The model under review builds one solid part; all positions refer to its coordinate system, in mm. Face numbers are marked on the shaded views. A direction names the side the tool comes from. Coordinates: 2 decimals unless noted, no trailing zeros. Write each loop counter-clockwise with the first axis right and the second up, starting at its lowest first coordinate (ties: lowest second). Pieces come first, ordered by that corner, then holes. Notation, with made-up numbers: M -38,66 L 13,66 A26 cw 13,101 Z; hole C -13,7.25 d8. An arc over 180 degrees is marked long. Answer as a JSON object with one key per item and string values.
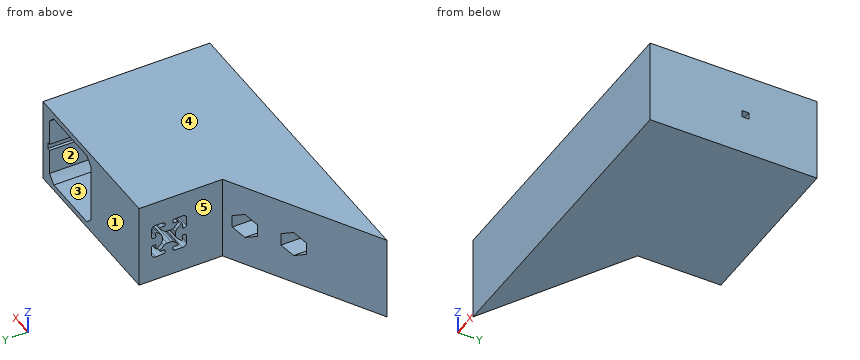
```python
from build123d import *

# Parameters (mm, degrees)
SKETCH1_W           = 35
SKETCH1_H           = 50
SKETCH1_W_2         = 62.5
BOSS_EXTRUDE1_DEPTH = 50
BOSS_EXTRUDE2_DEPTH = 50
CUT_EXTRUDE1_DEPTH  = 81
BOSS_EXTRUDE3_DEPTH = 50.006
SKETCH5_W           = 4
SKETCH5_H           = 4
CUT_EXTRUDE2_DEPTH  = 30
BOSS_EXTRUDE4_DEPTH = 50


with BuildPart() as part:
    # Sketch1 → Boss-Extrude1 (new body)
    # profile 1 of 2: a face of its own
    with BuildSketch(Plane.YZ):
        with Locations((80, 305)):
            Rectangle(SKETCH1_W, SKETCH1_H)
        with BuildLine():
            Line((76.1, 303.897755224), (76.1, 306.102244776))
            ThreePointArc((76.1, 306.102244776), (75.894474738, 307.135490044), (75.309188309, 308.011433085))
            Line((75.309188309, 308.011433085), (73.008308049, 310.312313346))
            ThreePointArc((73.008308049, 310.312313346), (72.488454457, 310.411010634), (72.206097787, 309.963502397))
            Line((72.206097787, 309.963502397), (72.280053987, 307.845673932))
            ThreePointArc((72.280053987, 307.845673932), (72.119231712, 307.415535218), (71.701359189, 307.225099738))
            Line((71.701359189, 307.225099738), (71.00178561, 307.20067009))
            ThreePointArc((71.00178561, 307.20067009), (70.213197967, 307.495510928), (69.864066254, 308.261610554))
            Line((69.864066254, 308.261610554), (69.701401098, 312.919731158))
            ThreePointArc((69.701401098, 312.919731158), (70.373654403, 314.626345597), (72.080268842, 315.298598902))
            Line((72.080268842, 315.298598902), (76.738389446, 315.135933746))
            ThreePointArc((76.738389446, 315.135933746), (77.504489072, 314.786802033), (77.79932991, 313.99821439))
            Line((77.79932991, 313.99821439), (77.774900262, 313.298640811))
            ThreePointArc((77.774900262, 313.298640811), (77.584464782, 312.880768288), (77.154326068, 312.719946013))
            Line((77.154326068, 312.719946013), (75.036497603, 312.793902213))
            ThreePointArc((75.036497603, 312.793902213), (74.588989366, 312.511545543), (74.687686654, 311.991691951))
            Line((74.687686654, 311.991691951), (76.988566915, 309.690811691))
            ThreePointArc((76.988566915, 309.690811691), (77.864509956, 309.105525262), (78.897755224, 308.9))
            Line((78.897755224, 308.9), (81.102244776, 308.9))
            ThreePointArc((81.102244776, 308.9), (82.135490044, 309.105525262), (83.011433085, 309.690811691))
            Line((83.011433085, 309.690811691), (85.312313346, 311.991691951))
            ThreePointArc((85.312313346, 311.991691951), (85.411010634, 312.511545543), (84.963502397, 312.793902213))
            Line((84.963502397, 312.793902213), (82.845673932, 312.719946013))
            ThreePointArc((82.845673932, 312.719946013), (82.415535218, 312.880768288), (82.225099738, 313.298640811))
            Line((82.225099738, 313.298640811), (82.20067009, 313.99821439))
            ThreePointArc((82.20067009, 313.99821439), (82.495510928, 314.786802033), (83.261610554, 315.135933746))
            Line((83.261610554, 315.135933746), (87.919731158, 315.298598902))
            ThreePointArc((87.919731158, 315.298598902), (89.626345597, 314.626345597), (90.298598902, 312.919731158))
            Line((90.298598902, 312.919731158), (90.135933746, 308.261610554))
            ThreePointArc((90.135933746, 308.261610554), (89.786802033, 307.495510928), (88.99821439, 307.20067009))
            Line((88.99821439, 307.20067009), (88.298640811, 307.225099738))
            ThreePointArc((88.298640811, 307.225099738), (87.880768288, 307.415535218), (87.719946013, 307.845673932))
            Line((87.719946013, 307.845673932), (87.793902213, 309.963502397))
            ThreePointArc((87.793902213, 309.963502397), (87.511545543, 310.411010634), (86.991691951, 310.312313346))
            Line((86.991691951, 310.312313346), (84.690811691, 308.011433085))
            ThreePointArc((84.690811691, 308.011433085), (84.105525262, 307.135490044), (83.9, 306.102244776))
            Line((83.9, 306.102244776), (83.9, 303.897755224))
            ThreePointArc((83.9, 303.897755224), (84.105525262, 302.864509956), (84.690811691, 301.988566915))
            Line((84.690811691, 301.988566915), (86.991691951, 299.687686654))
            ThreePointArc((86.991691951, 299.687686654), (87.511545543, 299.588989366), (87.793902213, 300.036497603))
            Line((87.793902213, 300.036497603), (87.719946013, 302.154326068))
            ThreePointArc((87.719946013, 302.154326068), (87.880768288, 302.584464782), (88.298640811, 302.774900262))
            Line((88.298640811, 302.774900262), (88.99821439, 302.79932991))
            ThreePointArc((88.99821439, 302.79932991), (89.786802033, 302.504489072), (90.135933746, 301.738389446))
            Line((90.135933746, 301.738389446), (90.298598902, 297.080268842))
            ThreePointArc((90.298598902, 297.080268842), (89.626345597, 295.373654403), (87.919731158, 294.701401098))
            Line((87.919731158, 294.701401098), (83.261610554, 294.864066254))
            ThreePointArc((83.261610554, 294.864066254), (82.495510928, 295.213197967), (82.20067009, 296.00178561))
            Line((82.20067009, 296.00178561), (82.225099738, 296.701359189))
            ThreePointArc((82.225099738, 296.701359189), (82.415535218, 297.119231712), (82.845673932, 297.280053987))
            Line((82.845673932, 297.280053987), (84.963502397, 297.206097787))
            ThreePointArc((84.963502397, 297.206097787), (85.411010634, 297.488454457), (85.312313346, 298.008308049))
            Line((85.312313346, 298.008308049), (83.011433085, 300.309188309))
            ThreePointArc((83.011433085, 300.309188309), (82.135490044, 300.894474738), (81.102244776, 301.1))
            Line((81.102244776, 301.1), (78.897755224, 301.1))
            ThreePointArc((78.897755224, 301.1), (77.864509956, 300.894474738), (76.988566915, 300.309188309))
            Line((76.988566915, 300.309188309), (74.687686654, 298.008308049))
            ThreePointArc((74.687686654, 298.008308049), (74.588989366, 297.488454457), (75.036497603, 297.206097787))
            Line((75.036497603, 297.206097787), (77.154326068, 297.280053987))
            ThreePointArc((77.154326068, 297.280053987), (77.584464782, 297.119231712), (77.774900262, 296.701359189))
            Line((77.774900262, 296.701359189), (77.79932991, 296.00178561))
            ThreePointArc((77.79932991, 296.00178561), (77.504489072, 295.213197967), (76.738389446, 294.864066254))
            Line((76.738389446, 294.864066254), (72.080268842, 294.701401098))
            ThreePointArc((72.080268842, 294.701401098), (70.373654403, 295.373654403), (69.701401098, 297.080268842))
            Line((69.701401098, 297.080268842), (69.864066254, 301.738389446))
            ThreePointArc((69.864066254, 301.738389446), (70.213197967, 302.504489072), (71.00178561, 302.79932991))
            Line((71.00178561, 302.79932991), (71.701359189, 302.774900262))
            ThreePointArc((71.701359189, 302.774900262), (72.119231712, 302.584464782), (72.280053987, 302.154326068))
            Line((72.280053987, 302.154326068), (72.206097787, 300.036497603))
            ThreePointArc((72.206097787, 300.036497603), (72.488454457, 299.588989366), (73.008308049, 299.687686654))
            Line((73.008308049, 299.687686654), (75.309188309, 301.988566915))
            ThreePointArc((75.309188309, 301.988566915), (75.894474738, 302.864509956), (76.1, 303.897755224))
        make_face(mode=Mode.SUBTRACT)
    # profile 2 of 2: a face of its own
    with BuildSketch(Plane.YZ):
        with Locations((31.25, 305)):
            Rectangle(SKETCH1_W_2, SKETCH1_H)
    extrude(amount=-BOSS_EXTRUDE1_DEPTH)

    # Sketch2 → Boss-Extrude2 (add)
    with BuildSketch(Plane(origin=(0, 0, 280), x_dir=(1, 0, 0), z_dir=(0, 0, -1))):
        Polygon((-50, -48.75), (-134.386033469, 0), (-50, 0), align=None)
    extrude(amount=-BOSS_EXTRUDE2_DEPTH)

    # Sketch3 → Cut-Extrude1 (cut)
    with BuildSketch(Plane(origin=(0, 97.5, 0), x_dir=(-1, 0, 0), z_dir=(0, 1, 0))):
        Polygon((67.990381057, 308.75), (61.495190528, 312.5), (55, 308.75), (55, 301.25), (61.495190528, 297.5), (67.990381057, 301.25), align=None)
        Polygon((92.990381057, 308.75), (86.495190528, 312.5), (80, 308.75), (80, 301.25), (86.495190528, 297.5), (92.990381057, 301.25), align=None)
    extrude(amount=-CUT_EXTRUDE1_DEPTH, mode=Mode.SUBTRACT)

    # Sketch4 → Boss-Extrude3 (add)
    with BuildSketch(Plane.XZ.offset(-47.494)):
        with BuildLine():
            Line((43.1, 322.104760785), (43.1, 306.85548466))
            Line((43.1, 306.85548466), (44.953275281, 306.85548466))
            Line((44.953275281, 306.85548466), (44.953275281, 302.922372887))
            Line((44.953275281, 302.922372887), (43.1, 302.922372887))
            Line((43.1, 302.922372887), (43.1, 287.895239215))
            ThreePointArc((43.1, 287.895239215), (41.005760925, 285.544239075), (38.654760785, 283.45))
            Line((38.654760785, 283.45), (4.445239215, 283.45))
            ThreePointArc((4.445239215, 283.45), (2.094239075, 285.544239075), (0, 287.895239215))
            Line((0, 287.895239215), (0, 280))
            Line((0, 280), (50, 280))
            Line((50, 280), (50, 330))
            Line((50, 330), (0, 330))
            Line((0, 330), (0, 322.104760785))
            ThreePointArc((0, 322.104760785), (2.094239075, 324.455760925), (4.445239215, 326.55))
            Line((4.445239215, 326.55), (38.654760785, 326.55))
            ThreePointArc((38.654760785, 326.55), (41.005760925, 324.455760925), (43.1, 322.104760785))
        make_face()
    extrude(amount=-BOSS_EXTRUDE3_DEPTH)

    # Sketch5 → Cut-Extrude2 (cut)
    with BuildSketch(Plane(origin=(44.953275281, 0, 0), x_dir=(0, -1, 0), z_dir=(-1, 0, 0))):
        with Locations((-55.75, 305)):
            Rectangle(SKETCH5_W, SKETCH5_H)
    extrude(amount=-CUT_EXTRUDE2_DEPTH, mode=Mode.SUBTRACT)

    # Sketch6 → Boss-Extrude4 (add)
    with BuildSketch(Plane.YZ):
        Polygon((0, 280), (47.494, 280), (47.494, 287.895239215), (47.494, 322.104760785), (47.494, 330), (0, 330), align=None)
    extrude(amount=BOSS_EXTRUDE4_DEPTH)


solid = part.part
```
(1) Add section D-D on y = 34.5. Give the boundary of the cut face in (x, z), and give its area (3 significant figures).
Results list:
{"outline": "M -74.67,280 L 50,280 L 50,330 L -74.67,330 Z; hole M -67.99,301.25 L -61.5,297.5 L -55,301.25 L -55,308.75 L -61.5,312.5 L -67.99,308.75 Z", "area": "6,090 mm²"}
(2) For pin 1 Ø5 at (y, z) = (37.5, 318.5) entering from -X; pin 2 Ø12 at (y, z) = (52, 313) entering from -X; pin 3 Ø24.5 at (y, z) = (84.5, 305.5) entering from -X, all flat-tipped, find the tip position at first contact; note any pin that passes through.
Results list:
{"pin 1": "x = -73.8", "pin 2": "x = -54.76", "pin 3": "x = -50"}
(3) Draft analysis for pull direction Z (two halves, no side actions). For the marked faces 3, 4 and 5, state which applies: released by +Z, released by -Z, zero draft, split by the parting line, or undercut.
Results list:
{"face 3": "undercut", "face 4": "released by +Z", "face 5": "zero draft"}
(4) Add section A-A on z = 319.5. Give the boundary of the cut face in (x, y).
Results list:
{"outline": "M -134.39,0 L 50,0 L 50,97.5 L 43.1,97.5 L 43.1,47.49 L 0,47.49 L 0,97.5 L -50,97.5 L -50,48.75 Z"}
(5) Add section B-B on y = 18.5. Give the boundary of the cut face in (x, z), and give its area (3 significant figures).
Results list:
{"outline": "M -102.36,280 L 50,280 L 50,330 L -102.36,330 Z; hole M -92.99,301.25 L -86.5,297.5 L -80,301.25 L -80,308.75 L -86.5,312.5 L -92.99,308.75 Z; hole M -67.99,301.25 L -61.5,297.5 L -55,301.25 L -55,308.75 L -61.5,312.5 L -67.99,308.75 Z", "area": "7,330 mm²"}
(6) For the marked faces 1 and 2, list the 3-axis set-ups (+Z, -Z, +X, -X, +Y, -Y) from which the entire face can be reached by the end or side of a thin tool; tool diameter is ignored.
Results list:
{"face 1": "+Z, -Z, +X, -X, +Y", "face 2": "+Y"}
(7) Wall thickness on line 1 along X through (y, z) = (65, 307); line 2 along Z through (x, y) = (22, 59); line 3 along Y through (x, z) = (-61.5, 296): over which ranges is each line inside the solid? List them lowest first. Write a range as from..to.
Results list:
{"line 1": "-50..0, 43.1..50", "line 2": "280..283.45, 326.55..330", "line 3": "0..42.11"}
(8) Add section C-C on x = 10.5. Give the boundary of the cut face in (y, z).
Results list:
{"outline": "M 0,280 L 97.5,280 L 97.5,283.45 L 47.49,283.45 L 47.49,326.55 L 97.5,326.55 L 97.5,330 L 0,330 Z"}
